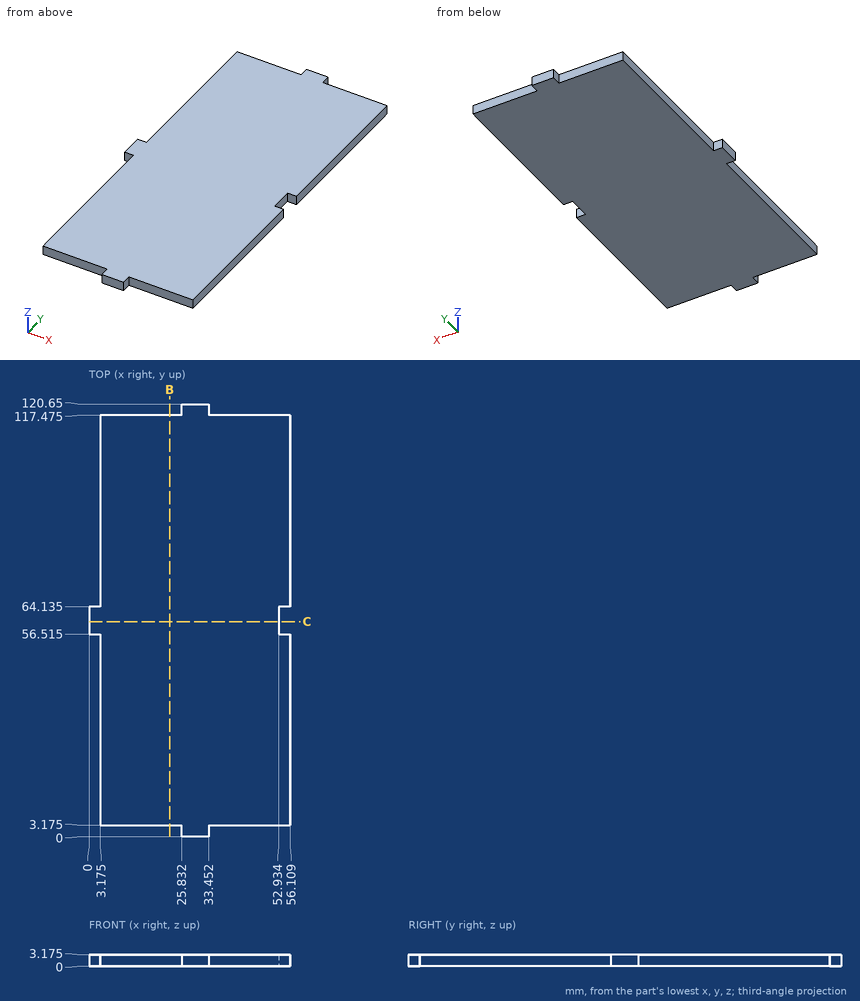
Design review of the part shown in the three views and the two pictorial views. Dimensions are in mm from the part's minimum x, y and z. Give positions to 0.01 mm unless a question says otherwise; leave off trailing zeros. Loops run counter-clockwise (first coordinate to the right, second up) from the corner with the lowest first, then second, coordinate; pieces in that order, holes last. Notation, with made-up numbers: M 2.25,68.25 L 42.25,68.25 A16 cw 42.25,97.25 Z; hole C 75.5,-7.5 d7. An arc over 180 degrees is marked long. Put each result on its own line as item: value. Start each with the question number.
(1) Add section B-B, the plane x = 22.5. Write out the cut boundary in (y, z) (1 decimal).
(2) For pin 1 (12 mm diameter, centred on x = 20, y = 91.5, fed in from -Z); pin 2 (1.6 mm diameter, centred on x = 2.5, z = 2.5, fed in from +Y) (3 decimals); pin 3 (1 mm diameter, centred on y = 2, z = 1.5, fed in from -X); pin 4 (1 mm diameter, centred on x = 48, z = 2, fed in from -Y) (3 decimals), all flat-tipped, find the tip position at first contact; note any pin that passes through.
(3) Wall thickness on L1, parallel to Y at x = 53, z = 0.7 (1 decimal); L2, parallel to Y at x = 13.5, z = 0.3 (1 decimal); L3, parallel to X at y = 64.5, z = 2.55 (1 decimal): over which ranges is each line inside the solid? List them lowest first.
(4) Add section C-C, the plane y = 60. Write out the cut boundary in (x, z) (1 decimal).
Result:
1. outline: M 3.2,0 L 117.5,0 L 117.5,3.2 L 3.2,3.2 Z
2. pin 1: stops at z = 0
2. pin 2: stops at y = 117.475
2. pin 3: stops at x = 25.83
2. pin 4: stops at y = 3.175
3. L1: y = 3.2 to 56.5, 64.1 to 117.5
3. L2: y = 3.2 to 117.5
3. L3: x = 3.2 to 56.1
4. outline: M 0,0 L 52.9,0 L 52.9,3.2 L 0,3.2 Z
